Verification items for the finished model (mm, model axes). Give positions to 0.01 mm unless a question says otherwise; leave off trailing zeros. Order: outer loops, then holes, each group sorted by start corner. A loop starts at its lowest first (then second) coordinate and runs counter-clockwise, first axis right, second up.
Autodesk Inventor part; units mm, degrees
ref_plane "YZ Plane" through (0, 0, 0) normal (1, 0, 0) x (0, 1, 0)
ref_plane "XZ Plane" through (0, 0, 0) normal (0, 1, 0) x (-1, 0, 0)
ref_plane "XY Plane" through (0, 0, 0) normal (0, 0, 1) x (1, 0, 0)
sketch "Sketch1" plane through (0, 0, 0) normal (0, 1, 0) x (-1, 0, 0)
  circle A0 centre (-94.6824, 281.0189) radius 1.4224
  circle A1 centre (-94.7479, 264.89) radius 1.4224
  circle A2 centre (-80.524, 264.8323) radius 1.4224
  circle A3 centre (-80.4585, 280.9611) radius 1.4224
  line L0 (-96.4532, 263.3256) -> (-77.4032, 263.3256) construction
  line L1 (-96.4532, 282.4506) -> (-96.4532, 263.4006) construction
  line L2 (-78.7132, 281.8156) -> (-96.4932, 281.8156)
  line L3 (-96.4932, 281.8156) -> (-96.4932, 264.0356)
  line L4 (-96.4932, 264.0356) -> (-78.7132, 264.0356)
  line L5 (-78.7132, 264.0356) -> (-78.7132, 281.8156)
  line L6 (-78.7132, 281.8156) -> (-96.4932, 264.0356) construction
  line L7 (-96.4932, 281.8156) -> (-78.7132, 264.0356) construction
  circle A4 centre (-87.6032, 272.9256) radius 2.5
  point P0 (0, 0)
extrude "Extrusion1" add sketch "Sketch1" along normal blind 3.175 contours A0 L2 A3 L5 L4 A2 A1 L3
(1) Section check D-D, the plane z = 272. Enter the section's corners in (x, y) (3 decimals), then the cut area to 3 significant figures.
Solved:
outline: (78.713, 0) - (85.281, 0) - (85.281, 3.175) - (78.713, 3.175) - close; (89.926, 0) - (96.493, 0) - (96.493, 3.175) - (89.926, 3.175) - close
area: 41.7 mm2
(2) Section check A-A, the plane z = 264.89. Give the number of separate pieces and of enclosed holes in the cut face, then the cut area to 3 significant figures.
Solved:
separate pieces: 3
enclosed holes: 0
area: 38.4 mm2
(3) Section check C-C, the plane y = 1.2. Enter the section's corners in (x, z), then the cut area to 3 significant figures.
Solved:
outline: (78.71, 264.04) - (79.35, 264.04) arc R1.42 cw (long way) to (81.7, 264.04) - (93.61, 264.04) arc R1.42 cw (long way) to (95.89, 264.04) - (96.49, 264.04) - (96.49, 281.82) - (95.86, 281.82) arc R1.42 cw (long way) to (93.5, 281.82) - (81.6, 281.82) arc R1.42 cw (long way) to (79.32, 281.82) - (78.71, 281.82) - close; hole circle Ø5 at (87.6, 272.93)
area: 275 mm2
(4) Section check B-B, the plane x = 87.25. Enter the section's corners in (y, z) (3 decimals), then the cut area to 3 significant figures.
Solved:
outline: (0, 264.036) - (3.175, 264.036) - (3.175, 270.451) - (0, 270.451) - close; (0, 275.401) - (3.175, 275.401) - (3.175, 281.816) - (0, 281.816) - close
area: 40.7 mm2
(5) Go/stop test with a flat-tipped pin: pin 1 (1.7 mm diameter, centred on x = 80.52, z = 264.83, fed in from +Y). Record where the tip stops, or that it passes through.
Solved:
pin 1: passes through
(6) Release check for a two-part mould opening along X. For faces 1 (the cylindrical face through (85.3, 1.6, 273.9)), 2 (the flat face through (87, 2, 281.816)), 3 (the flat face through (96.493, 2, 273)) record: pulls with the +X half, pulls with the -X half, needs draft (parallel to the pull), parting line crosses it, or undercut.
Solved:
face 1: undercut
face 2: needs draft
face 3: pulls with the +X half
(7) Scan lines: line 1 (Z direction, x = 87.5, y = 2.05); line 2 (X direction, y = 0.95, z = 265.25); line 3 (X direction, y = 0.75, z = 273). Record each from-to range of solid material in increasing order.
Solved:
line 1: z = 264.04 to 270.43, 275.42 to 281.82
line 2: x = 78.71 to 79.16, 81.88 to 93.37, 96.12 to 96.49
line 3: x = 78.71 to 85.1, 90.1 to 96.49
